Verification items for this drawing (mm, ordinates from the low corner). Round coordinates to 2 decimals unless told otherwise and drop trailing zeros. Order: outer loops, then holes, each group sorted by start corner. A loop starts at its lowest first (then second) coordinate and runs counter-clockwise, first axis right, second up. Notation, with made-up numbers: M 79,28 L 108,28 A21 cw 108,61 Z; hole C -21,7.5 d3. An arc over 180 degrees is marked long. One line per item, written item: value. Start each with the question number.
(1) Cross-section at A-A, the plane z = 1.75. Enter the section's corners in (x, y).
(2) Cross-section at C-C, the plane y = 9. Enter the section's corners in (x, z), and give its area (3 significant figures).
(3) Release check for a two-part mould opening along X. For the marked faces 1, 2, 3 and 4 record: released by +X, released by -X, zero draft, split by the parting line, or undercut.
(4) Thickness scan on L1, parallel to Y at x = 30, z = 3; L2, parallel to X at y = 37, z = 12; L3, parallel to Z at x = 10.5, y = 26.5. Record the ranges inside material, lowest first.
(5) Cross-section at B-B, the plane x = 30. Enter the section's corners in (y, z), and give its area (3 significant figures).
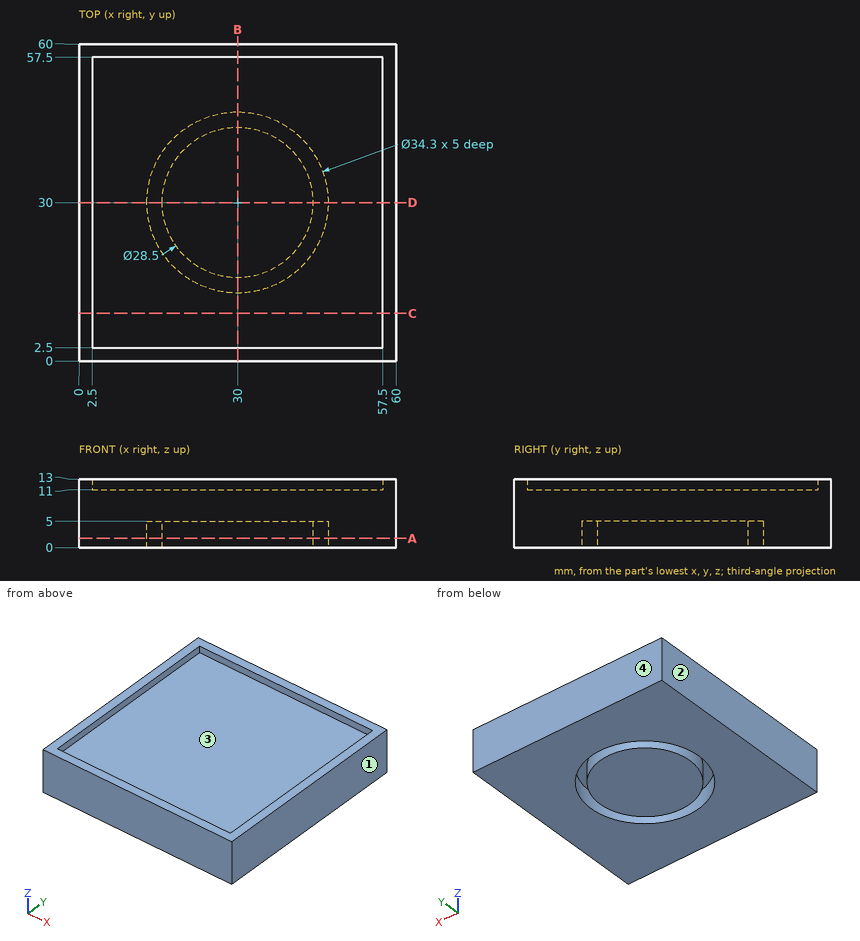
Values found:
1. outline: M 0,0 L 60,0 L 60,60 L 0,60 Z; C 30,30 d28.5; hole C 30,30 d34.3
2. outline: M 0,0 L 60,0 L 60,13 L 57.5,13 L 57.5,11 L 2.5,11 L 2.5,13 L 0,13 Z
2. area: 670 mm^2
3. face 1: released by +X
3. face 2: released by -X
3. face 3: undercut
3. face 4: zero draft
4. L1: 0 to 12.85, 15.75 to 44.25, 47.15 to 60
4. L2: 0 to 2.5, 57.5 to 60
4. L3: 0 to 11
5. outline: M 0,0 L 12.85,0 L 12.85,5 L 15.75,5 L 15.75,0 L 44.25,0 L 44.25,5 L 47.15,5 L 47.15,0 L 60,0 L 60,13 L 57.5,13 L 57.5,11 L 2.5,11 L 2.5,13 L 0,13 Z
5. area: 641 mm^2
